```python
from build123d import *

# Parameters (mm, degrees)
SKETCH1_W           = 77
SKETCH1_H           = 16
BOSS_EXTRUDE1_DEPTH = 2.8
SKETCH2_W           = 77
SKETCH2_H           = 8.24
BOSS_EXTRUDE2_DEPTH = 6.5
SKETCH4_W           = 3.18
SKETCH4_H           = 9.5
CUT_EXTRUDE1_DEPTH  = 10.3


with BuildPart() as part:
    # Sketch1 → Boss-Extrude1 (new body)
    with BuildSketch(Plane(origin=(0, 0, 0), x_dir=(1, 0, 0), z_dir=(0, 1, 0))):
        Rectangle(SKETCH1_W, SKETCH1_H)
    extrude(amount=BOSS_EXTRUDE1_DEPTH)

    # Sketch2 → Boss-Extrude2 (add)
    with BuildSketch(Plane(origin=(0, 2.8, 0), x_dir=(1, 0, 0), z_dir=(0, 1, 0))):
        Rectangle(SKETCH2_W, SKETCH2_H)
    extrude(amount=BOSS_EXTRUDE2_DEPTH)

    # Sketch4 → Cut-Extrude1 (cut, through all)
    with BuildSketch(Plane.XZ):
        with Locations((-26.95, 0)):
            Rectangle(SKETCH4_W, SKETCH4_H)
        with Locations((-34.65, 0)):
            Rectangle(SKETCH4_W, SKETCH4_H)
        with Locations((-19.25, 0)):
            Rectangle(SKETCH4_W, SKETCH4_H)
        with Locations((-11.55, 0)):
            Rectangle(SKETCH4_W, SKETCH4_H)
        with Locations((-3.85, 0)):
            Rectangle(SKETCH4_W, SKETCH4_H)
        with Locations((3.85, 0)):
            Rectangle(SKETCH4_W, SKETCH4_H)
        with Locations((11.55, 0)):
            Rectangle(SKETCH4_W, SKETCH4_H)
        with Locations((19.25, 0)):
            Rectangle(SKETCH4_W, SKETCH4_H)
        with Locations((26.95, 0)):
            Rectangle(SKETCH4_W, SKETCH4_H)
        with Locations((34.65, 0)):
            Rectangle(SKETCH4_W, SKETCH4_H)
    extrude(amount=-CUT_EXTRUDE1_DEPTH, mode=Mode.SUBTRACT)


solid = part.part
```
The model under review builds one solid part; all positions refer to its coordinate system, in mm. A direction names the side the tool comes from. Give positions to 0.01 mm unless a question says otherwise; leave off trailing zeros. Write each loop counter-clockwise with the first axis right and the second up, starting at its lowest first coordinate (ties: lowest second). Pieces come first, ordered by that corner, then holes.
(1) Tool access review of faces 1 (the flat face through (-31, 9.3, 0)), 2 (the flat face through (-1, 2.8, 6)), 3 (the flat face through (-17.66, 5, 0)), 4 (the flat face through (0, 6, -4.12)), 5 (the flat face through (-1, 0, 0)): name each direction out of +Z, -Z, +X, -X, +Y, -Y from which nothing blocks a thin tool from reaching the whole face with its end or side.
(2) Consider section A-A, the plane x = 27. Give the boundary of the cut face in (y, z), and give its area (3 significant figures).
(3) The part is to be moulded in two halves that separate along X. For faces 6 (the flat face through (35, 1, -4.75)), 7 (the flat face through (-8, 9.3, 0)), say which applies: released by +X, released by -X, zero draft, split by the parting line, or undercut.
(4) For P1, Ø1.4, axis at x = -1, y = 6, coming from the +Z side; P2, Ø4.5, axis at x = -15, z = 6.5, coming from the +Y side; P3, Ø2.5, axis at x = 22, y = 7.5, coming from the -Z side, all flat-tipped, find the tip position at first contact; note any pin that passes through.
(5) To check wall thickness, follow L1, parallel to Y at x = 7, z = -6.5; L2, parallel to Z at x = -14, y = 6.75. State the ranges of each line that lie inside material, in increasing order.
(6) Consider section B-B, the plane z = 0.5. Give the number of separate pieces and of enclosed holes in the cut face, and give its area (3 significant figures).
Returned:
1. face 1: +Z, -Z, +X, -X, +Y
1. face 2: +Z, +X, -X, +Y
1. face 3: +Y, -Y
1. face 4: -Z, +X, -X, +Y
1. face 5: +Z, -Z, +X, -X, -Y
2. outline: (0, -8) - (2.8, -8) - (2.8, -4.75) - (0, -4.75) - close; (0, 4.75) - (2.8, 4.75) - (2.8, 8) - (0, 8) - close
2. area: 18.2 mm2
3. face 6: undercut
3. face 7: zero draft
4. P1: stops at z = 4.12
4. P2: stops at y = 2.8
4. P3: stops at z = -4.12
5. L1: y = 0 to 2.8
5. L2: z = -4.12 to 4.12
6. separate pieces: 11
6. enclosed holes: 0
6. area: 420 mm2
